Source: CAD feature listing. Evaluate the final solid. Frame: model axes, mm. A direction names the side the tool comes from. Round coordinates to 2 decimals unless told otherwise and drop trailing zeros. Loops run counter-clockwise (first coordinate to the right, second up) from the corner with the lowest first, then second, coordinate; pieces in that order, holes last. Notation, with made-up numbers: (59.5, -22.5) -> (117.5, -22.5) arc R15 cw to (117.5, -2.5) -> close; hole circle Ø4 at (83.5, 60). An arc over 180 degrees is marked (long way). Write item = value, one per line.
Autodesk Inventor part; units mm, degrees
ref_plane "YZ Plane" through (0, 0, 0) normal (1, 0, 0) x (0, 1, 0)
ref_plane "XZ Plane" through (0, 0, 0) normal (0, 1, 0) x (-1, 0, 0)
ref_plane "XY Plane" through (0, 0, 0) normal (0, 0, 1) x (1, 0, 0)
sketch "Sketch1" plane through (0, 0, 0) normal (0, 1, 0) x (-1, 0, 0)
  circle A0 centre (0, 0) radius 30
  dimension "d0" = 60
extrude "Extrusion1" add sketch "Sketch1" along normal blind 3
sketch "Sketch2" plane through (0, 3, 0) normal (0, 1, 0) x (1, 0, 0)
  circle A0 centre (0, 0) radius 5
  dimension "d3" = 10
extrude "Extrusion2" cut sketch "Sketch2" against normal blind 4
sketch "Sketch4" plane through (0, 3, 0) normal (0, 1, 0) x (1, 0, 0)
  line L0 (-23.2158, -19.0158) -> (-11.2158, -19.0158)
  line L1 (-11.2158, -19.0158) -> (-11.2158, 10.9842)
  line L2 (-11.2158, 10.9842) -> (-23.2158, 10.9842)
  line L3 (-23.2158, 10.9842) -> (-23.2158, -19.0158)
  line L4 (-0.0289, -32.9889) -> (-0.0289, 43.4959) construction
  line L5 (23.1581, -19.0158) -> (11.1581, -19.0158)
  line L6 (11.1581, -19.0158) -> (11.1581, 10.9842)
  line L7 (11.1581, 10.9842) -> (23.1581, 10.9842)
  line L8 (23.1581, 10.9842) -> (23.1581, -19.0158)
  point P0 (0, -4.0158)
  point P1 (-23.2158, -4.0158)
  point P2 (23.2158, 0)
  dimension "d9" = 12
  dimension "d10" = 30
extrude "Extrusion4" add sketch "Sketch4" along normal blind 40
sketch "Sketch5" plane through (23.1581, 3, 19.0158) normal (1, 0, 0) x (0, 0, -1)
  line L0 (30, 0) -> (30, 40)
  line L1 (0, 0) -> (0, 40)
  arc A0 (30, 26.6004) -> (0, 26.7351) centre (14.9918, 24.8495) ccw
  line L2 (0, 26.7351) -> (0, 40)
  line L3 (30, 40) -> (0, 40)
  line L4 (30, 40) -> (30, 26.6004)
  point P0 (19.0158, -3)
extrude "Extrusion5" cut sketch "Sketch5" against normal blind 74.5
sketch "Sketch6" plane through (23.1581, 3, 19.0158) normal (1, 0, 0) x (0, 0, -1)
  circle A0 centre (15, 26.7283) radius 5.5
  point P0 (19.0158, -3)
  dimension "d15" = 11
extrude "Extrusion6" cut sketch "Sketch6" against normal blind 74.5
sketch "Sketch7" plane through (23.1581, 3, 19.0158) normal (1, 0, 0) x (0, 0, -1)
  line L0 (30, 0) -> (30, 26.6004)
  line L1 (30, 26.6004) -> (49.0158, 26.6004)
  line L2 (49.0158, 0) -> (-10.9842, 0)
  line L3 (49.0158, 26.6004) -> (49.0158, 0)
  point P0 (19.0158, -3)
  point P1 (0, 0)
  point P2 (0.0152, 0)
extrude "Extrusion7" add sketch "Sketch7" against normal blind 12
sketch "Sketch8" plane through (23.1581, 3, 19.0158) normal (1, 0, 0) x (0, 0, -1)
  circle A0 centre (39.1574, 13.257) radius 4.9
  point P0 (19.0158, -3)
  dimension "d20" = 9.8
extrude "Extrusion8" cut sketch "Sketch8" against normal blind 12
sketch "Sketch9" plane through (23.1581, 3, -30) normal (0, -1, 0) x (1, 0, 0)
  line L0 (-12, 0) -> (-12, 2.1522)
  arc A0 (-12, 2.1522) -> (0, 10.929) centre (-23.1581, 30) ccw
  arc A1 (-12, 2.1522) -> (0, 10.929) centre (-23.1408, 29.9763) ccw
  line L1 (0, 10.929) -> (0, 0)
  line L2 (0, 10.929) -> (0, 0)
  line L3 (0, 0) -> (-12, 0)
extrude "Extrusion9" cut sketch "Sketch9" against normal blind 33.25
fillet "Fillet1" radius 2 3 edges at (23.1581, 29.6004, -15.0276) (17.7109, 29.6004, -24.2152) (11.1581, 29.6004, -19.416)
sketch "Sketch10" plane through (-11.2158, 3, -10.9842) normal (0, 0, -1) x (-1, 0, 0)
  line L0 (0, 0) -> (0, 26.7351)
  line L1 (12, 0) -> (12, 26.7351)
  line L2 (0, 26.7351) -> (12, 26.7351)
  line L3 (12, 26.7351) -> (12, 0)
  line L4 (12, 0) -> (0, 0)
  line L5 (0, 0) -> (0, 26.7351)
  point P0 (-11.2158, -3)
extrude "Extrusion10" add sketch "Sketch10" along normal blind 5.656
sketch "Sketch11" plane through (-23.2158, 29.7351, -10.9842) normal (0, 1, 0) x (1, 0, 0)
  line L0 (12, -30) -> (12, 0)
  line L1 (0, -29.9848) -> (0, 5.656)
  line L2 (12, 0) -> (0, 0)
  line L3 (0, 0) -> (0, 5.656)
  line L4 (0, 5.656) -> (12, 5.656)
  line L5 (12, 5.656) -> (12, 0)
  point P0 (23.2158, -10.9842)
  point P1 (0, 0)
extrude "Extrusion11" add sketch "Sketch11" along normal blind 18
sketch "Sketch12" plane through (-23.2158, 3, 19.0158) normal (-1, 0, 0) x (0, 0, 1)
  line L0 (-30, 44.7351) -> (-30, 26.6004)
  line L1 (-30, 44.7351) -> (-14.9918, 44.7351)
  line L2 (-14.9918, 44.7351) -> (-14.9918, 39.9594)
  arc A0 (0, 26.7351) -> (-30.0997, 24.6004) centre (-14.9918, 24.8495) ccw
  point P0 (-19.0158, -3)
extrude "Extrusion12" add sketch "Sketch12" against normal blind 12
fillet "Fillet2" radius 5 1 edges at (-17.2158, 47.7351, 4.024)
sketch "Sketch13" plane through (-11.2158, 3, -16.6402) normal (0, 0, -1) x (-1, 0, 0)
  circle A0 centre (6.3211, 10.551) radius 1
  circle A1 centre (6.3211, 41.2302) radius 1
  point P0 (-11.2158, -3)
  dimension "d33" = 2
  dimension "d34" = 2
extrude "Extrusion13" cut sketch "Sketch13" against normal blind 14
sketch "Sketch15" plane through (0, 3, 0) normal (0, 1, 0) x (1, 0, 0)
  circle A0 centre (0, 0) radius 5
  circle A1 centre (0, 0) radius 10.5
  circle A2 centre (0, 0) radius 5
  dimension "d39" = 21
extrude "Extrusion15" add sketch "Sketch15" along normal blind 4
properties part number "base2_3DPrint"
1. Mould query, pull axis X, two halves, no side actions, for faces 1 (the face through (-16.8, 14.227, -9.738)), 2 (the face through (-23.216, 26, -3)), 3 (the face through (-17, 47.735, -9)). Classes: released by +X, released by -X, zero draft, split by the parting line, or undercut.
Evaluation:
face_1 = undercut
face_2 = released by -X
face_3 = zero draft
2. Line query: probe 1 along X at (y, z) = (4.5, -1); probe 2 along Z at (x, y) = (0, 3.25); probe 3 along X at (y, z) = (22, -4). Output: solid intervals per line, ascending. Write a range as from..to.
Evaluation:
probe_1 = -23.22..-11.22, -10.45..-4.9, 4.9..10.45, 11.16..23.16
probe_2 = -10.5..-5, 5..10.5
probe_3 = -23.22..-11.22, 11.16..23.16
3. Section query B-B (y = 31.5). Return the cut outline in (x, z).
Evaluation:
outline = (-23.22, -16.64) -> (-11.22, -16.64) -> (-11.22, -1.19) -> (-23.22, -1.19) -> close; (-23.22, 9.22) -> (-11.22, 9.22) -> (-11.22, 18.69) -> (-23.22, 18.69) -> close; (11.16, -10.64) -> (23.16, -10.64) -> (23.16, -1.19) -> (11.16, -1.19) -> close; (11.16, 9.22) -> (23.16, 9.22) -> (23.16, 18.69) -> (11.16, 18.69) -> close
4. Set-up query: faces 4 (the face through (10, 5, 3.2)), 5 (the face through (11.73, 29, -19.53)), 6 (the face through (15.909, 16.472, -15.246)), 7 (the face through (22.557, 29.03, -15.084)), 8 (the face through (5, 7, 2)). Return all of +Z, -Z, +X, -X, +Y, -Y with unobstructed straight access to the full face (end or side cutting, diameter ignored); none if empty.
Evaluation:
face_4 = +Y
face_5 = -Z, +Y
face_6 = +X
face_7 = -Z, +X, +Y
face_8 = +Z, -Z, +Y
5. Section query A-A (x = 0). Return the cut outline in (y, z), then the cut area to 3 significant figures.
Evaluation:
outline = (0, -30) -> (3, -30) -> (3, -10.5) -> (7, -10.5) -> (7, -5) -> (0, -5) -> close; (0, 5) -> (7, 5) -> (7, 10.5) -> (3, 10.5) -> (3, 30) -> (0, 30) -> close
area = 194 mm²
6. Section query D-D (x = -6.5). Return the cut outline in (y, z).
Evaluation:
outline = (0, -29.29) -> (3, -29.29) -> (3, -8.25) -> (7, -8.25) -> (7, 8.25) -> (3, 8.25) -> (3, 29.29) -> (0, 29.29) -> close
7. Section query C-C (z = 0). Return the cut outline in (x, y).
Evaluation:
outline = (-30, 0) -> (-5, 0) -> (-5, 7) -> (-10.5, 7) -> (-10.5, 3) -> (-11.22, 3) -> (-11.22, 25.97) -> (-23.22, 25.97) -> (-23.22, 3) -> (-30, 3) -> close; (-23.22, 33.49) -> (-11.22, 33.49) -> (-11.22, 47.64) -> (-23.22, 47.64) -> close; (5, 0) -> (30, 0) -> (30, 3) -> (23.16, 3) -> (23.16, 25.97) -> (11.16, 25.97) -> (11.16, 3) -> (10.5, 3) -> (10.5, 7) -> (5, 7) -> close; (11.16, 33.49) -> (23.16, 33.49) -> (23.16, 42.41) -> (11.16, 42.41) -> close
8. Contact query for flat-ended pins moving along their axis: pin 1 Ø6 at (x, y) = (-18.5, 38.5) entering from +Z; pin 2 Ø2.5 at (x, y) = (-17.54, 13.55) entering from -Z; pin 3 Ø8 at (y, z) = (16.26, -20.14) entering from +X. Output: stop coordinate, or through.
Evaluation:
pin_1 = 17.05
pin_2 = -16.64
pin_3 = -11.22
